Work out the finished part from the listing and answer in its coordinate system (mm). A direction names the side the tool comes from. Round coordinates to 2 decimals unless told otherwise and drop trailing zeros. Write each loop counter-clockwise with the first axis right and the second up, starting at its lowest first coordinate (ties: lowest second). Pieces come first, ordered by that corner, then holes.
1. A tool of negligible diameter and unlimited length cuts with its end or side. For faces 4 (the face through (-32, 0, 1)), 5 (the face through (-21, -21.07, 0.99)), from which of +Z, -Z, +X, -X, +Y, -Y can it reach the whole face along a straight path? Write none if from no direction.
2. A flat-ended cylindrical pin translates along its axis: pin 1 Ø5 at (x, y) = (-25, 30) entering from -Z. Find the tip coordinate at first contact, or state that the pin passes through.
3. Find section B-B (y = 30). Write down the section's boundary in (x, z).
4. Find section D-D (y = 4.5). Write down the section's boundary in (x, z), and give its area (3 significant figures).
5. Find section C-C (z = 1.15). Write down the section's boundary in (x, y).
6. Determine the mould class of faces 1 (the face through (0, -39.5, 1)), 2 (the face through (-30.57, -38, 1.01)), 3 (the face through (22.5, 0, 1)) for opening direction X: pulls with the +X half, pulls with the -X half, needs draft (parallel to the pull), parting line crosses it, or undercut.
7. Find section A-A (x = -25). Write down the section's boundary in (y, z), and give its area (3 significant figures).
8. Straight lines are drawn through the part: probe 1 along Y at (x, z) = (25, 1.3); probe 2 along X at (y, z) = (-30, 1.4); probe 3 along Y at (x, z) = (-17, 1.35). For each, find the intervals that lie inside material, in ascending order.
```python
from build123d import *

# Parameters (mm, degrees)
F0_W     = 64
F0_H     = 79
F0_W_2   = 50
F0_H_2   = 60
F1_DEPTH = 2
F2_D     = 6
F3_R     = 5
F4_W     = 45
F4_H     = 45
F5_DEPTH = 25
F6_R     = 5


with BuildPart() as f1:
    # F0 (on Top) → F1 (new body)
    with BuildSketch(Plane.XY):
        Rectangle(F0_W, F0_H)
        Rectangle(F0_W_2, F0_H_2, mode=Mode.SUBTRACT)
        Rectangle(F0_W_2, F0_H_2)
    extrude(amount=F1_DEPTH)

    # F2 (through all)
    with Locations(Plane(origin=(0, 0, 0), x_dir=(1, 0, 0), z_dir=(0, 0, -1))):
        with Locations((25, 30), (-25, 30), (-25, -30), (25, -30)):
            Hole(F2_D / 2)

    # F3
    f3_edges = [f1.edges().sort_by_distance(p)[0] for p in [
        (-32, -39.5, 1),
        (32, -39.5, 1),
        (-32, 39.5, 1),
        (32, 39.5, 1),
    ]]
    fillet(f3_edges, radius=F3_R)

    # F4 (on face) → F5 (cut)
    with BuildSketch(Plane.XY.offset(2)):
        Rectangle(F4_W, F4_H)
    extrude(amount=-F5_DEPTH, mode=Mode.SUBTRACT)

    # F6
    f6_edges = [f1.edges().sort_by_distance(p)[0] for p in [
        (-22.5, 22.5, 1),
        (22.5, 22.5, 1),
        (22.5, -22.5, 1),
        (-22.5, -22.5, 1),
    ]]
    fillet(f6_edges, radius=F6_R)


solid = f1.part
```
Worked answers:
1. face 4: +Z, -Z, -X, +Y, -Y
1. face 5: +Z, -Z
2. pin 1: passes through
3. outline: (-32, 0) - (-28, 0) - (-28, 2) - (-32, 2) - close; (-22, 0) - (22, 0) - (22, 2) - (-22, 2) - close; (28, 0) - (32, 0) - (32, 2) - (28, 2) - close
4. outline: (-32, 0) - (-22.5, 0) - (-22.5, 2) - (-32, 2) - close; (22.5, 0) - (32, 0) - (32, 2) - (22.5, 2) - close
4. area: 38.0 mm2
5. outline: (-32, -34.5) arc R5 ccw to (-27, -39.5) - (27, -39.5) arc R5 ccw to (32, -34.5) - (32, 34.5) arc R5 ccw to (27, 39.5) - (-27, 39.5) arc R5 ccw to (-32, 34.5) - close; hole circle Ø6 at (-25, -30); hole circle Ø6 at (-25, 30); hole (-22.5, -17.5) arc R5 ccw to (-17.5, -22.5) - (17.5, -22.5) arc R5 ccw to (22.5, -17.5) - (22.5, 17.5) arc R5 ccw to (17.5, 22.5) - (-17.5, 22.5) arc R5 ccw to (-22.5, 17.5) - close; hole circle Ø6 at (25, -30); hole circle Ø6 at (25, 30)
6. face 1: needs draft
6. face 2: pulls with the -X half
6. face 3: undercut
7. outline: (-39.5, 0) - (-33, 0) - (-33, 2) - (-39.5, 2) - close; (-27, 0) - (27, 0) - (27, 2) - (-27, 2) - close; (33, 0) - (39.5, 0) - (39.5, 2) - (33, 2) - close
7. area: 134 mm2
8. probe 1: y = -39.5 to -33, -27 to 27, 33 to 39.5
8. probe 2: x = -32 to -28, -22 to 22, 28 to 32
8. probe 3: y = -39.5 to -22.5, 22.5 to 39.5
